```python
from build123d import *

# Parameters (mm, degrees)
F0_R     = 9.4
F1_DEPTH = 3


with BuildPart() as f1:
    # F0 (on Front) → F1 (new body)
    with BuildSketch(Plane.XZ):
        with BuildLine():
            Line((58.8, 11.4), (0, 11.4))
            ThreePointArc((0, 11.4), (-9.870808, 5.703258), (-9.87645, -5.693483))
            Line((-9.87645, -5.693483), (-0.07645, -22.693483))
            Line((-0.07645, -22.693483), (19.523115, -56.692727))
            Line((19.523115, -56.692727), (29.322897, -73.692349))
            ThreePointArc((29.322897, -73.692349), (33.496089, -77.869674), (39.199347, -79.398866))
            Line((39.199347, -79.398866), (176.399347, -79.398866))
            ThreePointArc((176.399347, -79.398866), (186.270155, -73.702124), (186.275796, -62.305384))
            Line((186.275796, -62.305384), (176.476014, -45.305762))
            Line((176.476014, -45.305762), (147.07645, 5.693483))
            ThreePointArc((147.07645, 5.693483), (142.903258, 9.870808), (137.2, 11.4))
            Line((137.2, 11.4), (98, 11.4))
            Line((98, 11.4), (58.8, 11.4))
        make_face()
        with Locations((39.199347, -67.998866)):
            Circle(F0_R, mode=Mode.SUBTRACT)
        with Locations((58.799347, -67.998866)):
            Circle(F0_R, mode=Mode.SUBTRACT)
        with Locations((78.399347, -67.998866)):
            Circle(F0_R, mode=Mode.SUBTRACT)
        with Locations((29.399564, -50.999244)):
            Circle(F0_R, mode=Mode.SUBTRACT)
        with Locations((19.599782, -33.999622)):
            Circle(F0_R, mode=Mode.SUBTRACT)
        with Locations((48.999564, -50.999244)):
            Circle(F0_R, mode=Mode.SUBTRACT)
        with Locations((68.599564, -50.999244)):
            Circle(F0_R, mode=Mode.SUBTRACT)
        with Locations((88.199564, -50.999244)):
            Circle(F0_R, mode=Mode.SUBTRACT)
        with Locations((39.199782, -33.999622)):
            Circle(F0_R, mode=Mode.SUBTRACT)
        with Locations((58.799782, -33.999622)):
            Circle(F0_R, mode=Mode.SUBTRACT)
        with Locations((78.399782, -33.999622)):
            Circle(F0_R, mode=Mode.SUBTRACT)
        with Locations((97.999347, -67.998866)):
            Circle(F0_R, mode=Mode.SUBTRACT)
        with Locations((117.599347, -67.998866)):
            Circle(F0_R, mode=Mode.SUBTRACT)
        with Locations((137.199347, -67.998866)):
            Circle(F0_R, mode=Mode.SUBTRACT)
        with Locations((156.799347, -67.998866)):
            Circle(F0_R, mode=Mode.SUBTRACT)
        with Locations((176.399347, -67.998866)):
            Circle(F0_R, mode=Mode.SUBTRACT)
        with Locations((107.799564, -50.999244)):
            Circle(F0_R, mode=Mode.SUBTRACT)
        with Locations((127.399564, -50.999244)):
            Circle(F0_R, mode=Mode.SUBTRACT)
        with Locations((97.999782, -33.999622)):
            Circle(F0_R, mode=Mode.SUBTRACT)
        with Locations((117.599782, -33.999622)):
            Circle(F0_R, mode=Mode.SUBTRACT)
        with Locations((137.199782, -33.999622)):
            Circle(F0_R, mode=Mode.SUBTRACT)
        with Locations((146.999564, -50.999244)):
            Circle(F0_R, mode=Mode.SUBTRACT)
        with Locations((166.599564, -50.999244)):
            Circle(F0_R, mode=Mode.SUBTRACT)
        with Locations((156.799782, -33.999622)):
            Circle(F0_R, mode=Mode.SUBTRACT)
        with BuildLine():
            ThreePointArc((9.8, -26.4), (5.097314, -25.139087), (1.656261, -21.694626))
            ThreePointArc((1.656261, -21.694626), (7.370097, -7.919495), (19.2, -17))
            ThreePointArc((19.2, -17), (16.446804, -23.646804), (9.8, -26.4))
        make_face(mode=Mode.SUBTRACT)
        with Locations((29.4, -17)):
            Circle(F0_R, mode=Mode.SUBTRACT)
        with Locations((49, -17)):
            Circle(F0_R, mode=Mode.SUBTRACT)
        with BuildLine():
            ThreePointArc((76.743739, -12.305374), (77.680505, -14.570097), (78, -17))
            ThreePointArc((78, -17), (75.246804, -23.646804), (68.6, -26.4))
            ThreePointArc((68.6, -26.4), (60.460913, -12.297314), (76.743739, -12.305374))
        make_face(mode=Mode.SUBTRACT)
        with BuildLine():
            ThreePointArc((0, 9.4), (6.646804, 6.646804), (9.4, 0))
            ThreePointArc((9.4, 0), (2.429903, -9.080505), (-8.143739, -4.694626))
            ThreePointArc((-8.143739, -4.694626), (-8.139087, 4.702686), (0, 9.4))
        make_face(mode=Mode.SUBTRACT)
        with BuildLine():
            ThreePointArc((29, 0), (12.953196, -6.646804), (19.6, 9.4))
            ThreePointArc((19.6, 9.4), (26.246804, 6.646804), (29, 0))
        make_face(mode=Mode.SUBTRACT)
        with BuildLine():
            ThreePointArc((48.6, 0), (32.553196, -6.646804), (39.2, 9.4))
            ThreePointArc((39.2, 9.4), (45.846804, 6.646804), (48.6, 0))
        make_face(mode=Mode.SUBTRACT)
        with BuildLine():
            ThreePointArc((68.2, 0), (52.153196, -6.646804), (58.8, 9.4))
            ThreePointArc((58.8, 9.4), (63.502686, 8.139087), (66.943739, 4.694626))
            ThreePointArc((66.943739, 4.694626), (67.880505, 2.429903), (68.2, 0))
        make_face(mode=Mode.SUBTRACT)
        with Locations((78.4, 0)):
            Circle(F0_R, mode=Mode.SUBTRACT)
        with Locations((88.2, -17)):
            Circle(F0_R, mode=Mode.SUBTRACT)
        with Locations((107.8, -17)):
            Circle(F0_R, mode=Mode.SUBTRACT)
        with Locations((127.4, -17)):
            Circle(F0_R, mode=Mode.SUBTRACT)
        with Locations((147, -17)):
            Circle(F0_R, mode=Mode.SUBTRACT)
        with Locations((98, 0)):
            Circle(F0_R, mode=Mode.SUBTRACT)
        with Locations((117.6, 0)):
            Circle(F0_R, mode=Mode.SUBTRACT)
        with Locations((137.2, 0)):
            Circle(F0_R, mode=Mode.SUBTRACT)
    extrude(amount=F1_DEPTH)


solid = f1.part
```
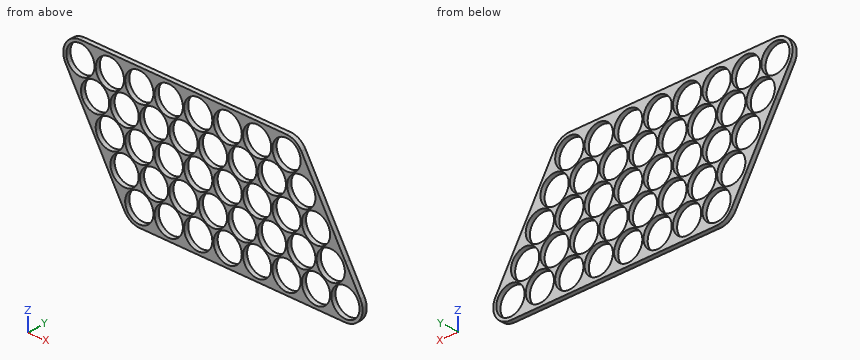
The listing builds one solid part. Answer for the finished solid, in the listing's coordinates (mm). Give positions to 0.01 mm unless a question says otherwise; leave off trailing zeros. Order: outer loops, then holes, each group sorted by start corner. A loop starts at its lowest first (then second) coordinate and runs counter-clockwise, first axis right, second up.
Item 1: Find the intervals of material crossed by probe 1 along Z at (x, y) = (137.2, -1.45); probe 2 along Z at (x, y) = (49, -2.1); probe 3 along Z at (x, y) = (112, -1.9), in increasing order.
From the geometry:
probe 1: z = -79.4 to -77.4, -58.6 to -43.4, -24.6 to -9.4, 9.4 to 11.4
probe 2: z = -79.4 to -60.4, -41.6 to -26.4, -7.6 to 11.4
probe 3: z = -79.4 to -75.55, -60.45 to -59.41, -42.59 to -41.55, -26.45 to -25.41, -8.59 to -7.55, 7.55 to 11.4
Item 2: The part is cut by section D-D, the plane x = 54. Give the vertices of the cut face in (y, z).
From the geometry:
outline: (-3, -79.4) - (0, -79.4) - (0, -76.08) - (-3, -76.08) - close; (-3, -59.92) - (0, -59.92) - (0, -58.96) - (-3, -58.96) - close; (-3, -43.04) - (0, -43.04) - (0, -42.08) - (-3, -42.08) - close; (-3, -25.92) - (0, -25.92) - (0, -24.96) - (-3, -24.96) - close; (-3, -9.04) - (0, -9.04) - (0, -8.08) - (-3, -8.08) - close; (-3, 8.08) - (0, 8.08) - (0, 11.4) - (-3, 11.4) - close
Item 3: The part is cut by section B-B, the plane z = -31.5. Count the separate pieces of the cut face and the enclosed holes in it, and give its area (3 significant figures).
From the geometry:
separate pieces: 9
enclosed holes: 0
area: 55.6 mm2
Item 4: Given pin 1 Ø1 at (x, z) = (163, -44) entering from +Y, flat-ended and moving along its own axis, determine where the tip first touches the part or whether it passes through.
From the geometry:
pin 1: passes through
Item 5: The part is cut by section A-A, the plane x = 123. Give the vertices of the cut face in (y, z).
From the geometry:
outline: (-3, -79.4) - (0, -79.4) - (0, -75.69) - (-3, -75.69) - close; (-3, -60.31) - (0, -60.31) - (0, -59.31) - (-3, -59.31) - close; (-3, -42.69) - (0, -42.69) - (0, -41.69) - (-3, -41.69) - close; (-3, -26.31) - (0, -26.31) - (0, -25.31) - (-3, -25.31) - close; (-3, -8.69) - (0, -8.69) - (0, -7.69) - (-3, -7.69) - close; (-3, 7.69) - (0, 7.69) - (0, 11.4) - (-3, 11.4) - close
